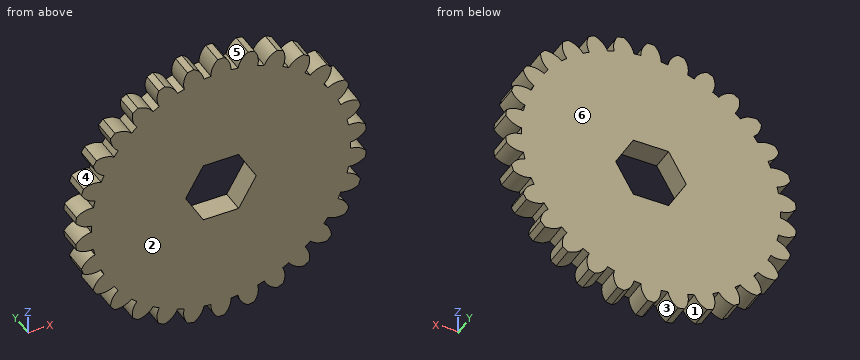
from build123d import *

# Parameters (mm, degrees)
SKETCH2_R           = 26.923711167
BOSS_EXTRUDE2_DEPTH = 4.7625
BOSS_EXTRUDE3_DEPTH = 4.7625
CIRPATTERN1_COUNT   = 30


with BuildPart() as part:
    # Sketch2 → Boss-Extrude2 (new body)
    with BuildSketch(Plane(origin=(0, 0, 0), x_dir=(1, 0, 0), z_dir=(0, 1, 0))):
        Circle(SKETCH2_R)
        Polygon((7.332348419, 0), (3.666174209, 6.35), (-3.666174209, 6.35), (-7.332348419, 0), (-3.666174209, -6.35), (3.666174209, -6.35), align=None, mode=Mode.SUBTRACT)
    extrude(amount=BOSS_EXTRUDE2_DEPTH)

    # Sketch1 → Boss-Extrude3 (add)
    with BuildSketch(Plane(origin=(0, 0, 0), x_dir=(1, 0, 0), z_dir=(0, 1, 0))):
        with BuildLine():
            Line((0.673251408, 30.249487652), (-0.673251408, 30.249487652))
            ThreePointArc((-0.673251408, 30.249487652), (-1.756386228, 28.702610818), (-2.084301351, 26.842911743))
            ThreePointArc((-2.084301351, 26.842911743), (0, 26.923711167), (2.084301351, 26.842911743))
            ThreePointArc((2.084301351, 26.842911743), (1.756386228, 28.702610818), (0.673251408, 30.249487652))
        make_face()
    boss_extrude3 = extrude(amount=BOSS_EXTRUDE3_DEPTH)

    # CirPattern1: Boss-Extrude3 ×30 about axis
    cirpattern1_axis = Axis((0, 0, 0), (0, 1, 0))
    for i in range(1, CIRPATTERN1_COUNT):
        add(boss_extrude3.rotate(cirpattern1_axis, i * 360 / CIRPATTERN1_COUNT))


solid = part.part
Geometry: final body of the model. Coordinates: model frame, mm. Face numbers are marked on the shaded views. A direction names the side the tool comes from. Give positions to 0.01 mm unless a question says otherwise; leave off trailing zeros. Loops run counter-clockwise (first coordinate to the right, second up) from the corner with the lowest first, then second, coordinate; pieces in that order, holes last. Notation, with made-up numbers: M 49.5,28.25 L 65.5,28.25 A10 ccw 65.5,45.25 Z; hole C -11,-23 d5. An arc over 180 degrees is marked long. Put each result on its own line as item: value. Start each with the question number.
1) Contact query for a flat-ended pin moving along its axis: pin 1 (2 mm diameter, centred on y = 2, z = -7, fed in from -X). Output: stop coordinate, or through.
2) Cut plane A-A (z = -1.5). Output: boundary loops of the cut face in (x, y), then the cut area to 3 significant figures.
3) Access query for the marked faces 4, 5 and 6. Directions: +Z, -Z, +X, -X, +Y, -Y. A direction counts if a zero-diameter tool reaches every point of the face in a straight line with its end or side. Return the directions, or none.
4) Cut plane C-C (z = -18.5). Output: boundary loops of the cut face in (x, y).
5) Cut plane B-B (x = -15.5). Output: boundary loops of the cut face in (y, z), then the cut area to 3 significant figures.
6) Ray query, line 1 along Z through (x, y) = (27, 1.1); line 2 along X through (y, z) = (0.2, 0); line 3 along X through (y, z) = (1.7, -12). Return the intervals inside material, ascending.
7) Pull-direction query (X, two-part tool) for the marked faces 1, 2 and 3; classes: pulls with the +X half, pulls with the -X half, needs draft (parallel to the pull), parting line crosses it, or undercut.
Verdict:
1. pin 1: x = -28.57
2. outline: M -29.13,0 L -6.47,0 L -6.47,4.76 L -29.13,4.76 Z; M 6.47,0 L 29.13,0 L 29.13,4.76 L 6.47,4.76 Z
2. area: 216 mm2
3. face 4: +Y, -Y
3. face 5: +Z, +Y, -Y
3. face 6: +Z, -Z, +X, -X, +Y
4. outline: M -22.74,0 L 22.74,0 L 22.74,4.76 L -22.74,4.76 Z
5. outline: M 0,-24.28 L 4.76,-24.28 L 4.76,24.28 L 0,24.28 Z
5. area: 231 mm2
6. line 1: -10.51 to -6.64, -4.92 to -0.74, 0.74 to 4.92, 6.64 to 10.51
6. line 2: -26.92 to -7.33, 7.33 to 26.92
6. line 3: -24.9 to 24.9
7. face 1: undercut
7. face 2: needs draft
7. face 3: undercut
